Can you work these out from the model? Positions are in its coordinate system, mm. Round coordinates to 2 decimals unless told otherwise and drop trailing zeros. Order: outer loops, then holes, each group sorted by start corner. A loop starts at its lowest first (then second) coordinate and runs counter-clockwise, first axis right, second up.
Q1. Will these pins go through, and if not, where does the flat tip stop? P1, Ø15, axis at x = -186.5, y = 0, coming from the -Z side; P2, Ø15, axis at x = 173.5, z = -20, coming from the +Y side; P3, Ø8.5, axis at x = 425, z = -20, coming from the -Y side.
Q2. If we section it at C-C (y = 13): Please give me the cut outline in (x, z), plus the area to 3 significant figures.
Q3. If we section it at B-B (x = 75): Please give me the cut outline in (y, z), plus the area to 3 significant figures.
Q4. If we section it at A-A (z = -31): Please give me the cut outline in (x, y), plus the area to 3 significant figures.
Q5. If I drill on line 1 (Z direction, x = -173.5, y = 36.25); line 2 (Y direction, x = 186, z = -4); line 3 (Y direction, x = -233, z = -14), over which ranges is the centre line in solid material (lowest first)?
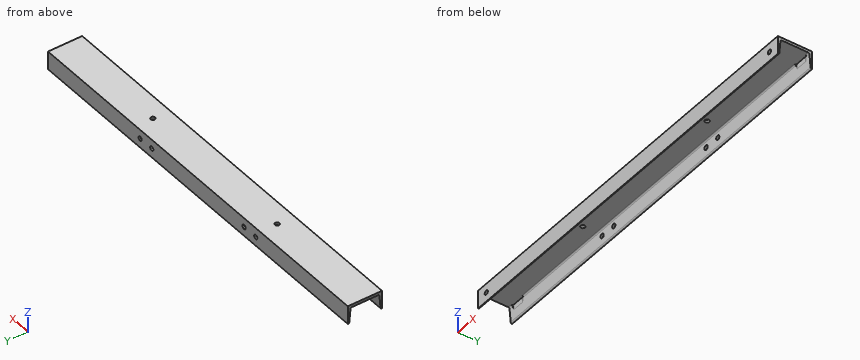
from build123d import *

# Parameters (mm, degrees)
STRUCTURAL_MEMBER1_DEPTH = 900
SKETCH12_R               = 4.7625
CUT_EXTRUDE1_DEPTH       = 454.327971782
CUT_EXTRUDE2_DEPTH       = 40
SKETCH16_R               = 4.7625
CUT_EXTRUDE3_DEPTH       = 454.327971881
SKETCH17_R               = 4.7625
CUT_EXTRUDE4_DEPTH       = 454.327971881


with BuildPart() as part:
    # Sketch19 → Structural Member1 (new body)
    with BuildSketch(Plane(origin=(-450, 0, 0), x_dir=(0, 0, 1), z_dir=(1, 0, 0))):
        with BuildLine():
            Line((0, 37.5), (0, -37.5))
            Line((0, -37.5), (-40, -37.5))
            Line((-40, -37.5), (-40, -37.246949676))
            ThreePointArc((-40, -37.246949676), (-39.212582687, -35.220998578), (-37.263681431, -34.258560126))
            Line((-37.263681431, -34.258560126), (-8.736318569, -31.741439874))
            ThreePointArc((-8.736318569, -31.741439874), (-6.787417313, -30.779001422), (-6, -28.753050324))
            Line((-6, -28.753050324), (-6, 28.753050324))
            ThreePointArc((-6, 28.753050324), (-6.787417313, 30.779001422), (-8.736318569, 31.741439874))
            Line((-8.736318569, 31.741439874), (-37.263681431, 34.258560126))
            ThreePointArc((-37.263681431, 34.258560126), (-39.212582687, 35.220998578), (-40, 37.246949676))
            Line((-40, 37.246949676), (-40, 37.5))
            Line((-40, 37.5), (0, 37.5))
        make_face()
    extrude(amount=STRUCTURAL_MEMBER1_DEPTH)

    # Sketch12 → Cut-Extrude1 (cut, through all)
    with BuildSketch(Plane(origin=(0, 0, 0), x_dir=(1, 0, 0), z_dir=(0, 1, 0))):
        with Locations(Location((-425, 20, 0), (0, 0, 270))):
            Circle(SKETCH12_R)
        with Locations(Location((425, 20, 0), (0, 0, 270))):
            Circle(SKETCH12_R)
    extrude(amount=-CUT_EXTRUDE1_DEPTH, mode=Mode.SUBTRACT)

    # Sketch15 → Cut-Extrude2 (cut)
    with BuildSketch(Plane(origin=(0, 0, -6), x_dir=(-1, 0, 0), z_dir=(0, 0, -1))):
        with BuildLine():
            Line((-412.5, 22.5), (-437.5, 22.5))
            ThreePointArc((-437.5, 22.5), (-442.5, 27.5), (-437.5, 32.5))
            Line((-437.5, 32.5), (-412.5, 32.5))
            ThreePointArc((-412.5, 32.5), (-407.5, 27.5), (-412.5, 22.5))
        make_face()
        with BuildLine():
            Line((412.5, 22.5), (437.5, 22.5))
            ThreePointArc((437.5, 22.5), (442.5, 27.5), (437.5, 32.5))
            Line((437.5, 32.5), (412.5, 32.5))
            ThreePointArc((412.5, 32.5), (407.5, 27.5), (412.5, 22.5))
        make_face()
    extrude(amount=CUT_EXTRUDE2_DEPTH, mode=Mode.SUBTRACT)

    # Sketch16 → Cut-Extrude3 (cut, through all)
    with BuildSketch(Plane(origin=(0, 0, 0), x_dir=(1, 0, 0), z_dir=(0, 1, 0))):
        with Locations(Location((-173.5, 20, 0), (0, 0, 270))):
            Circle(SKETCH16_R)
        with Locations(Location((-138.5, 20, 0), (0, 0, 270))):
            Circle(SKETCH16_R)
        with Locations(Location((138.5, 20, 0), (0, 0, 90))):
            Circle(SKETCH16_R)
        with Locations(Location((173.5, 20, 0), (0, 0, 90))):
            Circle(SKETCH16_R)
    extrude(amount=CUT_EXTRUDE3_DEPTH, mode=Mode.SUBTRACT)

    # Sketch17 → Cut-Extrude4 (cut, through all)
    with BuildSketch(Plane.XY):
        with Locations((-186.5, 0)):
            Circle(SKETCH17_R)
        with Locations((186.5, 0)):
            Circle(SKETCH17_R)
    extrude(amount=-CUT_EXTRUDE4_DEPTH, mode=Mode.SUBTRACT)


solid = part.part
Solution:
1. P1: stops at z = -6
1. P2: stops at y = 37.5
1. P3: stops at y = 32.5
2. outline: (-450, -6) - (450, -6) - (450, 0) - (-450, 0) - close
2. area: 5,400 mm2
3. outline: (-37.5, -40) - (-37.25, -40) arc R3 ccw to (-34.26, -37.26) - (-31.74, -8.74) arc R3 cw to (-28.75, -6) - (28.75, -6) arc R3 cw to (31.74, -8.74) - (34.26, -37.26) arc R3 ccw to (37.25, -40) - (37.5, -40) - (37.5, 0) - (-37.5, 0) - close
3. area: 756 mm2
4. outline: (-450, -37.5) - (450, -37.5) - (450, -33.71) - (-450, -33.71) - close; (-450, 33.71) - (450, 33.71) - (450, 37.5) - (-450, 37.5) - close
4. area: 6,830 mm2
5. line 1: z = -39.83 to -24.76, -15.24 to 0
5. line 2: y = -37.5 to -4.74, 4.74 to 37.5
5. line 3: y = -37.5 to -32.21, 32.21 to 37.5
